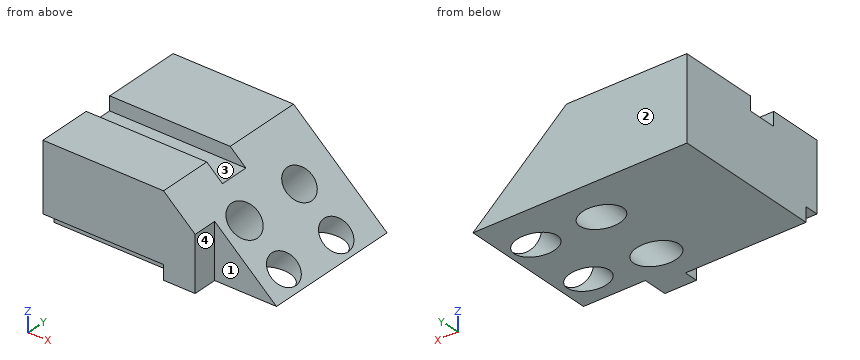
from build123d import *

# Parameters (mm, degrees)
F0_W      = 65.9222155809
F0_H      = 45.1669357717
F1_DEPTH  = 76.2
F2_W      = 65.9222155809
F2_H      = 16.1303170025
F3_DEPTH  = 7.62
F5_DEPTH  = 13.462
F6_W      = 51.6149867326
F6_H      = 45.1669357717
F7_DEPTH  = 13.462
F8_W      = 65.9222155809
F8_H      = 7.957983762
F9_DEPTH  = 7.62
F10_DEPTH = 25.4
F11_R     = 9.3419450296
F11_R_2   = 8.7268718577
F11_R_3   = 8.921818007
F11_R_4   = 8.8708982801
F12_DEPTH = 88.646


with BuildPart() as f1:
    # F0 (on Front) → F1 (new body)
    with BuildSketch(Plane.XZ):
        with Locations((-32.9611077905, 22.5834678859)):
            Rectangle(F0_W, F0_H)
        Polygon((0, 45.1669357717), (0, 0), (51.0816499591, 0), align=None)
    extrude(amount=F1_DEPTH)

    # F2 (on face) → F3 (cut)
    with BuildSketch(Plane.XY.offset(45.1669357717)):
        with Locations((-32.9611077905, -51.7781917006)):
            Rectangle(F2_W, F2_H)
    extrude(amount=-F3_DEPTH, mode=Mode.SUBTRACT)

    # F4 (on face) → F5 (join)
    with BuildSketch(Plane.XZ.offset(76.2)):
        Polygon((17.2973467296, 0), (17.2973467296, 29.8724386405), (0, 45.1669357717), (-14.3072288483, 45.1669357717), (-14.3072288483, 0), align=None)
    extrude(amount=F5_DEPTH)

    # F6 (on face) → F7 (join)
    with BuildSketch(Plane.XZ.offset(76.2)):
        with Locations((-40.1147222146, 22.5834678859)):
            Rectangle(F6_W, F6_H)
    extrude(amount=F7_DEPTH)

    # F8 (on face) → F9 (cut)
    with BuildSketch(Plane.XZ.offset(89.662)):
        with Locations((-32.9611077905, 3.978991881)):
            Rectangle(F8_W, F8_H)
    extrude(amount=-F9_DEPTH, mode=Mode.SUBTRACT)

    # F10 (cut): a face of the model
    f10_faces = [f1.faces().sort_by_distance(p)[0] for p in [
        (0, -51.7781917006, 41.3569357717),
    ]]
    extrude(f10_faces, amount=-F10_DEPTH, mode=Mode.SUBTRACT)

    # F11 (on face) → F12 (cut)
    with BuildSketch(Plane(origin=(22.4135408595, 0, 25.348645618), x_dir=(0.7491470366, 0, -0.6624037421), z_dir=(0.6624037421, 0, 0.7491470366))):
        with Locations((0, -62.0419606566)):
            Circle(F11_R)
        with Locations((26.7226807773, -60.1655058563)):
            Circle(F11_R_2)
        with Locations((0, -24.1914074868)):
            Circle(F11_R_3)
        with Locations((26.9680060446, -24.3262052536)):
            Circle(F11_R_4)
    extrude(amount=-F12_DEPTH, mode=Mode.SUBTRACT)


solid = f1.part
The listing builds one solid part. Answer for the finished solid, in the listing's coordinates (mm). Face numbers are marked on the shaded views. Round coordinates to 2 decimals unless told otherwise and drop trailing zeros. Order: outer loops, then holes, each group sorted by start corner. A loop starts at its lowest first (then second) coordinate and runs counter-clockwise, first axis right, second up. Notation, with made-up numbers: (78.25, -23.75) -> (123.25, -23.75) arc R19 cw to (123.25, 0.25) -> close; hole circle Ø10 at (-16, 28). An arc over 180 degrees is marked (long way). One line per item, written item: value.
Item 1: Given P1, Ø2.5, axis at y = -85.5, z = 4.5, coming from the -X side; P2, Ø4, axis at y = -13.5, z = 22.5, coming from the +X side; P3, Ø12, axis at x = -12.5, z = 22.5, coming from the +Y side; P4, Ø2.5, axis at x = -39.5, z = 5.5, coming from the -Y side, each flat-ended and moving along its own axis, determine where each tip first touches the part or whether it passes through.
Taken from the geometry:
P1: stops at x = 0
P2: stops at x = 27.9
P3: stops at y = 0
P4: stops at y = -82.04
Item 2: For a pull along Y with two mould halves and no side action, classify the marked faces 1, 2, 3 and 4 as released by +Y, released by -Y, zero draft, split by the parting line, or undercut.
Taken from the geometry:
face 1: released by -Y
face 2: released by +Y
face 3: undercut
face 4: zero draft
Item 3: Find section A-A, the plane y = -57. Give the vertices of the cut face in (x, z).
Taken from the geometry:
outline: (-65.92, 0) -> (-10.5, 0) -> (16.52, 30.56) -> (8.62, 37.55) -> (-65.92, 37.55) -> close; (10.5, 0) -> (24.82, 0) -> (36.34, 13.03) -> (28.31, 20.14) -> close; (46.53, 0) -> (51.08, 0) -> (48.53, 2.26) -> close
Item 4: Find section C-C, the plane x = 39. State how many separate pieces and enclosed holes the cut face has, then the cut area to 3 significant figures.
Taken from the geometry:
separate pieces: 3
enclosed holes: 0
area: 452 mm2
Item 5: Find section B-B, the plane x = -16. Give the vertices of the cut face in (y, z).
Taken from the geometry:
outline: (-89.66, 7.96) -> (-82.04, 7.96) -> (-82.04, 0) -> (0, 0) -> (0, 45.17) -> (-43.71, 45.17) -> (-43.71, 37.55) -> (-59.84, 37.55) -> (-59.84, 45.17) -> (-89.66, 45.17) -> close
Item 6: Straight lines are drawn through the part: L1, parallel to Y at x = -13.5, z = 41; L2, parallel to Y at x = 33, z = 12; L3, parallel to Y at x = 10, z = 8. For each, find the intervals that lie inside material, in ascending order.
Taken from the geometry:
L1: y = -89.66 to -59.84, -43.71 to 0
L2: y = -76.2 to 0
L3: y = -89.66 to -71.12, -52.96 to -32.84, -15.54 to 0
